from build123d import *

# Parameters (mm, degrees)
SKETCH_1_R          = 1.5
SKETCH_1_R_2        = 2.5
EXTRUDE_1_DEPTH     = 5
CUT_EXTRUDE_1_DEPTH = 167.58331249
FILLET_1_R          = 3


with BuildPart() as part:
    # 草图1 → 凸台-拉伸1 (new body)
    with BuildSketch(Plane(origin=(0, 0, 0), x_dir=(1, 0, 0), z_dir=(0, 1, 0))):
        with BuildLine():
            Line((-125, 85), (-67.999242617, 85))
            ThreePointArc((-67.999242617, 85), (-64.463708711, 86.464466094), (-62.999242617, 90))
            Line((-62.999242617, 90), (-62.999242617, 105))
            ThreePointArc((-62.999242617, 105), (-61.534776523, 108.535533906), (-57.999242617, 110))
            Line((-57.999242617, 110), (-37.999242617, 110))
            ThreePointArc((-37.999242617, 110), (-34.463708711, 108.535533906), (-32.999242617, 105))
            Line((-32.999242617, 105), (-32.999242617, 90))
            ThreePointArc((-32.999242617, 90), (-31.534776523, 86.464466094), (-27.999242617, 85))
            Line((-27.999242617, 85), (49.000757383, 85))
            Line((49.000757383, 85), (49.000757383, -85))
            Line((49.000757383, -85), (-27.999242617, -85))
            ThreePointArc((-27.999242617, -85), (-31.534776523, -86.464466094), (-32.999242617, -90))
            Line((-32.999242617, -90), (-32.999242617, -105))
            ThreePointArc((-32.999242617, -105), (-34.463708711, -108.535533906), (-37.999242617, -110))
            Line((-37.999242617, -110), (-57.999242617, -110))
            ThreePointArc((-57.999242617, -110), (-61.534776523, -108.535533906), (-62.999242617, -105))
            Line((-62.999242617, -105), (-62.999242617, -90))
            ThreePointArc((-62.999242617, -90), (-64.463708711, -86.464466094), (-67.999242617, -85))
            Line((-67.999242617, -85), (-125, -85))
            Line((-125, -85), (-125, -46.78057254))
            Line((-125, -46.78057254), (-102.434615997, -46.78057254))
            Line((-102.434615997, -46.78057254), (-102.434615997, 46.78057254))
            Line((-102.434615997, 46.78057254), (-125, 46.78057254))
            Line((-125, 46.78057254), (-125, 85))
        make_face()
        with Locations(Location((-120.84, -82.25, 0), (0, 0, 270))):
            Circle(SKETCH_1_R, mode=Mode.SUBTRACT)
        with Locations(Location((-110.34, -82.25, 0), (0, 0, 270))):
            Circle(SKETCH_1_R, mode=Mode.SUBTRACT)
        with Locations(Location((-81.34, -82.25, 0), (0, 0, 270))):
            Circle(SKETCH_1_R, mode=Mode.SUBTRACT)
        with Locations(Location((-81.34, 82.25, 0), (0, 0, 90))):
            Circle(SKETCH_1_R, mode=Mode.SUBTRACT)
        with Locations(Location((-110.34, 82.25, 0), (0, 0, 90))):
            Circle(SKETCH_1_R, mode=Mode.SUBTRACT)
        with Locations(Location((-120.84, 82.25, 0), (0, 0, 90))):
            Circle(SKETCH_1_R, mode=Mode.SUBTRACT)
        with Locations(Location((6.16, 82.25, 0), (0, 0, 90))):
            Circle(SKETCH_1_R, mode=Mode.SUBTRACT)
        with Locations(Location((16.66, 82.25, 0), (0, 0, 90))):
            Circle(SKETCH_1_R, mode=Mode.SUBTRACT)
        with Locations(Location((45.66, 82.25, 0), (0, 0, 90))):
            Circle(SKETCH_1_R, mode=Mode.SUBTRACT)
        with Locations(Location((6.16, -82.25, 0), (0, 0, 270))):
            Circle(SKETCH_1_R, mode=Mode.SUBTRACT)
        with Locations(Location((16.66, -82.25, 0), (0, 0, 270))):
            Circle(SKETCH_1_R, mode=Mode.SUBTRACT)
        with Locations(Location((45.66, -82.25, 0), (0, 0, 270))):
            Circle(SKETCH_1_R, mode=Mode.SUBTRACT)
        with Locations(Location((-69.422345539, 28.355497102, 0), (0, 0, 270))):
            Circle(SKETCH_1_R_2, mode=Mode.SUBTRACT)
        with Locations(Location((0.577654461, 28.355497102, 0), (0, 0, 270))):
            Circle(SKETCH_1_R_2, mode=Mode.SUBTRACT)
        with Locations(Location((-69.422345539, -19.644502898, 0), (0, 0, 270))):
            Circle(SKETCH_1_R_2, mode=Mode.SUBTRACT)
        with Locations(Location((0.577654461, -19.644502898, 0), (0, 0, 270))):
            Circle(SKETCH_1_R_2, mode=Mode.SUBTRACT)
        with Locations(Location((-59.249242617, -106.1, 0), (0, 0, 270))):
            Circle(SKETCH_1_R, mode=Mode.SUBTRACT)
        with Locations(Location((-36.749242617, -106.1, 0), (0, 0, 90))):
            Circle(SKETCH_1_R, mode=Mode.SUBTRACT)
        with Locations(Location((-47.999242617, -97.789393477, 0), (0, 0, 270))):
            Circle(SKETCH_1_R, mode=Mode.SUBTRACT)
        with Locations(Location((-36.749242617, 106.1, 0), (0, 0, 270))):
            Circle(SKETCH_1_R, mode=Mode.SUBTRACT)
        with Locations(Location((-59.249242617, 106.1, 0), (0, 0, 90))):
            Circle(SKETCH_1_R, mode=Mode.SUBTRACT)
        with Locations(Location((-47.999242617, 97.789393477, 0), (0, 0, 90))):
            Circle(SKETCH_1_R, mode=Mode.SUBTRACT)
        with BuildLine():
            Line((-12.914937196, -51.31082178), (-83.083548039, -51.31082178))
            ThreePointArc((-83.083548039, -51.31082178), (-90.154615851, -54.239753968), (-93.083548039, -61.31082178))
            Line((-93.083548039, -61.31082178), (-93.083548039, -61.770331604))
            ThreePointArc((-93.083548039, -61.770331604), (-90.154615851, -68.841399416), (-83.083548039, -71.770331604))
            Line((-83.083548039, -71.770331604), (-12.914937196, -71.770331604))
            ThreePointArc((-12.914937196, -71.770331604), (-5.843869384, -68.841399416), (-2.914937196, -61.770331604))
            Line((-2.914937196, -61.770331604), (-2.914937196, -61.31082178))
            ThreePointArc((-2.914937196, -61.31082178), (-5.843869384, -54.239753968), (-12.914937196, -51.31082178))
        make_face(mode=Mode.SUBTRACT)
        with BuildLine():
            Line((-12.914937196, 71.770331604), (-83.083548039, 71.770331604))
            ThreePointArc((-83.083548039, 71.770331604), (-90.154615851, 68.841399416), (-93.083548039, 61.770331604))
            Line((-93.083548039, 61.770331604), (-93.083548039, 61.31082178))
            ThreePointArc((-93.083548039, 61.31082178), (-90.154615851, 54.239753968), (-83.083548039, 51.31082178))
            Line((-83.083548039, 51.31082178), (-12.914937196, 51.31082178))
            ThreePointArc((-12.914937196, 51.31082178), (-5.843869384, 54.239753968), (-2.914937196, 61.31082178))
            Line((-2.914937196, 61.31082178), (-2.914937196, 61.770331604))
            ThreePointArc((-2.914937196, 61.770331604), (-5.843869384, 68.841399416), (-12.914937196, 71.770331604))
        make_face(mode=Mode.SUBTRACT)
        with BuildLine():
            Line((-15.665960641, 45.130463402), (-54.200019018, 45.130463402))
            ThreePointArc((-54.200019018, 45.130463402), (-61.27108683, 42.201531214), (-64.200019018, 35.130463402))
            Line((-64.200019018, 35.130463402), (-64.200019018, -35.130463402))
            ThreePointArc((-64.200019018, -35.130463402), (-61.27108683, -42.201531214), (-54.200019018, -45.130463402))
            Line((-54.200019018, -45.130463402), (-15.665960641, -45.130463402))
            ThreePointArc((-15.665960641, -45.130463402), (-8.594892829, -42.201531214), (-5.665960641, -35.130463402))
            Line((-5.665960641, -35.130463402), (-5.665960641, 35.130463402))
            ThreePointArc((-5.665960641, 35.130463402), (-8.594892829, 42.201531214), (-15.665960641, 45.130463402))
        make_face(mode=Mode.SUBTRACT)
    extrude(amount=EXTRUDE_1_DEPTH)

    # 草图2 → 切除-拉伸1 (cut, through all)
    with BuildSketch(Plane.XZ):
        with BuildLine():
            Line((21.556311208, 45.130463402), (38.464260393, 45.130463402))
            ThreePointArc((38.464260393, 45.130463402), (41.999794299, 43.665997308), (43.464260393, 40.130463402))
            Line((43.464260393, 40.130463402), (43.464260393, -40.130463402))
            ThreePointArc((43.464260393, -40.130463402), (41.999794299, -43.665997308), (38.464260393, -45.130463402))
            Line((38.464260393, -45.130463402), (21.556311208, -45.130463402))
            ThreePointArc((21.556311208, -45.130463402), (18.020777302, -43.665997308), (16.556311208, -40.130463402))
            Line((16.556311208, -40.130463402), (16.556311208, 40.130463402))
            ThreePointArc((16.556311208, 40.130463402), (18.020777302, 43.665997308), (21.556311208, 45.130463402))
        make_face()
    extrude(amount=-CUT_EXTRUDE_1_DEPTH, mode=Mode.SUBTRACT)

    # 圆角1
    fillet_1_edges = [part.edges().sort_by_distance(p)[0] for p in [
        (-125, 2.5, 46.78057254),
        (-102.434615997, 2.5, 46.78057254),
        (-102.434615997, 2.5, -46.78057254),
        (-125, 2.5, -46.78057254),
    ]]
    fillet(fillet_1_edges, radius=FILLET_1_R)


solid = part.part
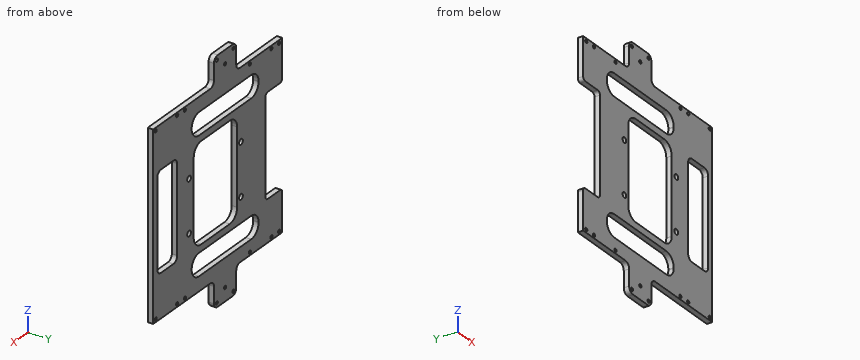
CAD build for the part. Positions are in the model's coordinates, mm. Give positions to 0.01 mm unless a question says otherwise; leave off trailing zeros. Write each loop counter-clockwise with the first axis right and the second up, starting at its lowest first coordinate (ties: lowest second). Pieces come first, ordered by that corner, then holes. Notation, with made-up numbers: (-6, -39.75) -> (11, -39.75) arc R21 ccw to (11, -5.75) -> close; hole circle Ø5 at (4, 1.25). An arc over 180 degrees is marked (long way). Return JSON: item names as keys, results as strings.
Item 1: Drill centre lines: probe 1 along Z at (x, y) = (-50, 4.4); probe 2 along X at (y, z) = (1.4, -5); probe 3 along Z at (x, y) = (-81.34, 1.35). Where is each one in solid material? Low to high.
Answer below:
{"probe 1": "z = -110 to -71.77, -51.31 to -45.13, 45.13 to 51.31, 71.77 to 110", "probe 2": "x = -102.43 to -64.2, -5.67 to 16.56, 43.46 to 49", "probe 3": "z = -85 to -83.75, -80.75 to -71.77, -51.31 to 51.31, 71.77 to 80.75, 83.75 to 85"}
Item 2: Drop flat-ended pins along their axis: pin 1 (2.5 mm diameter, centred on x = 6.16, z = 82.25, fed in from -Y); pin 2 (1.5 mm diameter, centred on x = -37, y = 3.5, fed in from -Z); pin 3 (1.5 mm diameter, centred on y = 1.5, z = -2.5, fed in from -X); pin 4 (3 mm diameter, centred on x = 10.5, y = 0.5, fed in from -Z). Give the stop position or say it passes through.
Answer below:
{"pin 1": "passes through", "pin 2": "stops at z = -109.99", "pin 3": "stops at x = -102.43", "pin 4": "stops at z = -85"}
Item 3: Band-saw the part on A-A (x = 11). List the corners of the cut face in (y, z).
Answer below:
{"outline": "(0, -85) -> (5, -85) -> (5, 85) -> (0, 85) -> close"}
Item 4: Band-saw the part on B-B (y = 1). Give the number of separate pieces and of enclosed holes in the cut face, then the cut area to 3 significant figures.
Answer below:
{"separate pieces": "1", "enclosed holes": "26", "area": "17,600 mm2"}
